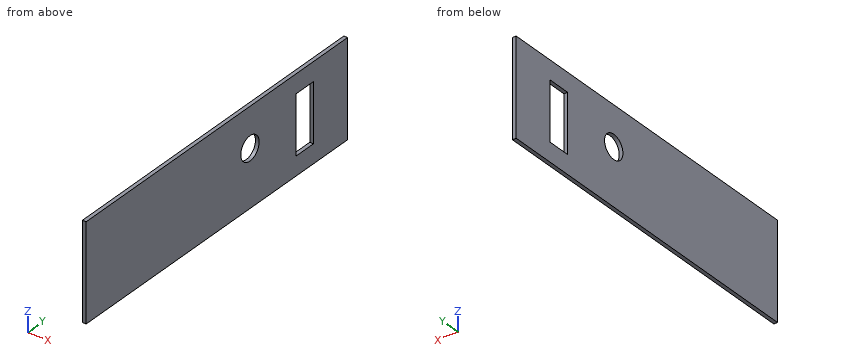
from build123d import *

# Parameters (mm, degrees)
SKETCH1_W           = 82.55
SKETCH1_H           = 292.1
BOSS_EXTRUDE1_DEPTH = 3.175
CUT_EXTRUDE1_REACH  = 305.557
SKETCH2_W           = 50.25
SKETCH2_H           = 19.5
CUT_EXTRUDE2_REACH  = 305.557
SKETCH4_R           = 10.25


with BuildPart() as part:
    # Sketch1 → Boss-Extrude1 (new body)
    with BuildSketch(Plane(origin=(0, 0, 0), x_dir=(0, 0, -1), z_dir=(1, 0, 0))):
        with Locations((41.275, 146.05)):
            Rectangle(SKETCH1_W, SKETCH1_H)
    extrude(amount=BOSS_EXTRUDE1_DEPTH)

    # Sketch2 → Cut-Extrude1 (cut, up to next)
    with BuildSketch(Plane.ZY, mode=Mode.PRIVATE) as cut_extrude1_sk1:
        with Locations((-41.275, 244.25)):
            Rectangle(SKETCH2_W, SKETCH2_H)
    cut_extrude1_tool1 = extrude(cut_extrude1_sk1.sketch, amount=-CUT_EXTRUDE1_REACH, mode=Mode.PRIVATE) & part.part
    add(cut_extrude1_tool1.solids().sort_by_distance((0, 244.25, -41.275))[0], mode=Mode.SUBTRACT)

    # Sketch4 → Cut-Extrude2 (cut, up to next)
    with BuildSketch(Plane.ZY, mode=Mode.PRIVATE) as cut_extrude2_sk1:
        with Locations((-33.963522547, 183.037474176)):
            Circle(SKETCH4_R)
    cut_extrude2_tool1 = extrude(cut_extrude2_sk1.sketch, amount=-CUT_EXTRUDE2_REACH, mode=Mode.PRIVATE) & part.part
    add(cut_extrude2_tool1.solids().sort_by_distance((0, 183.037474, -33.963523))[0], mode=Mode.SUBTRACT)


solid = part.part
The model under review builds one solid part; all positions refer to its coordinate system, in mm. Round coordinates to 2 decimals unless told otherwise and drop trailing zeros. Loops run counter-clockwise (first coordinate to the right, second up) from the corner with the lowest first, then second, coordinate; pieces in that order, holes last. Notation, with made-up numbers: (5.25, 13.5) - (42.25, 13.5) arc R21 ccw to (42.25, 21.5) - close; hole circle Ø10 at (79.5, 17). An arc over 180 degrees is marked (long way). Use CSV: the item, a comma, the result in double quotes.
(1) Take a section at C-C, the plane x = 0.85. Give the boundary of the cut face in (y, z), plus the area to 3 significant figures.
Working result:
outline,"(0, -82.55) - (292.1, -82.55) - (292.1, 0) - (0, 0) - close; hole circle Ø20.5 at (183.04, -33.96); hole (234.5, -66.4) - (254, -66.4) - (254, -16.15) - (234.5, -16.15) - close"
area,"22,800 mm^2"
(2) Take a section at A-A, the plane y = 238. Give the boundary of the cut face in (x, z) (3 decimals).
Working result:
outline,"(0, -82.55) - (3.175, -82.55) - (3.175, -66.4) - (0, -66.4) - close; (0, -16.15) - (3.175, -16.15) - (3.175, 0) - (0, 0) - close"
(3) Take a section at B-B, the plane z = -50. Give the boundary of the cut face in (x, y) (3 decimals), plus the area to 3 significant figures.
Working result:
outline,"(0, 0) - (3.175, 0) - (3.175, 234.5) - (0, 234.5) - close; (0, 254) - (3.175, 254) - (3.175, 292.1) - (0, 292.1) - close"
area,"866 mm^2"
(4) For line 1 (Y direction, x = 1.4, z = -22); line 2 (Y direction, x = 2.5, z = -38.5); line 3 (Y direction, x = 2.9, z = -24.5), list the stretches that pass through material, from the lowest coordinate up.
Working result:
line 1,"y = 0 to 234.5, 254 to 292.1"
line 2,"y = 0 to 173.85, 192.23 to 234.5, 254 to 292.1"
line 3,"y = 0 to 179.1, 186.98 to 234.5, 254 to 292.1"
